```python
from build123d import *

# Parameters (mm, degrees)
F0_R     = 3.2639
F0_R_2   = 14.224
F1_DEPTH = 12.7
F2_R     = 6.35


# Not quite as in the source:
# - ends of sketch curves that miss each other by under 0.0002 mm in the source are joined


with BuildPart() as f1:
    # F0 (on Top) → F1 (new body)
    with BuildSketch(Plane.XY):
        with BuildLine():
            Line((-19.0499999385, -12.7), (19.0500000615, -12.7))
            ThreePointArc((19.0500000615, -12.7), (23.5401281437, -10.8401280388), (25.4000000615, -6.3499999385))
            Line((25.4000000615, -6.3499999385), (25.3999998771, 12.7))
            Line((25.3999998771, 12.7), (20.257849715, 41.692909813))
            ThreePointArc((20.257849715, 41.692909813), (0, 58.674), (-20.257849715, 41.692909813))
            Line((-20.257849715, 41.692909813), (-25.4000001229, 12.7))
            Line((-25.4000001229, 12.7), (-25.3999999385, -6.3500000615))
            ThreePointArc((-25.3999999385, -6.3500000615), (-23.5401279774, -10.8401280823), (-19.0499999385, -12.7))
        make_face()
        with Locations((-16.256, 0)):
            Circle(F0_R, mode=Mode.SUBTRACT)
        with Locations((15.494, 0)):
            Circle(F0_R, mode=Mode.SUBTRACT)
        with Locations((0, 38.1)):
            Circle(F0_R_2, mode=Mode.SUBTRACT)
    extrude(amount=F1_DEPTH)

    # F2
    f2_edges = [f1.edges().sort_by_distance(p)[0] for p in [
        (25.4, 12.7, 6.35),
        (-25.4, 12.7, 6.35),
    ]]
    fillet(f2_edges, radius=F2_R)


solid = f1.part
```
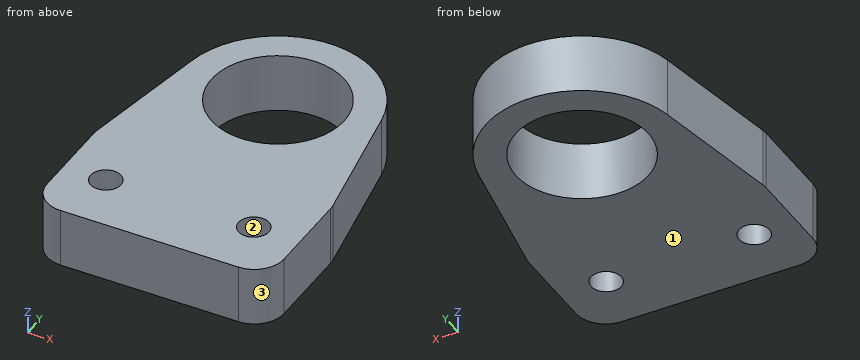
Part model, mm, in its own coordinate system. Face numbers are marked on the shaded views. Round coordinates to 2 decimals unless told otherwise and drop trailing zeros. Write each loop counter-clockwise with the first axis right and the second up, starting at its lowest first coordinate (ties: lowest second). Pieces come first, ordered by that corner, then holes.
Item 1: Probe L1, parallel to X at y = -1, z = 2.25; L2, parallel to Y at x = 0, z = 5.25; L3, parallel to X at y = 49, z = 12. List the from-to ranges inside material, lowest first.
Results:
L1: x = -25.4 to -19.36, -13.15 to 12.39, 18.6 to 25.4
L2: y = -12.7 to 23.88, 52.32 to 58.67
L3: x = -17.45 to -9.14, 9.14 to 17.45
Item 2: Cut at B-B, the plane x = 0. Give the cut face in (y, z).
Results:
outline: (-12.7, 0) - (23.88, 0) - (23.88, 12.7) - (-12.7, 12.7) - close; (52.32, 0) - (58.67, 0) - (58.67, 12.7) - (52.32, 12.7) - close
Item 3: Cut at C-C, the plane z = 6.5. Give the cut face in (x, y).
Results:
outline: (-25.4, -6.35) arc R6.35 ccw to (-19.05, -12.7) - (19.05, -12.7) arc R6.35 ccw to (25.4, -6.35) - (25.4, 12.14) arc R6.35 ccw to (25.3, 13.25) - (20.26, 41.69) arc R20.57 ccw to (-20.26, 41.69) - (-25.3, 13.25) arc R6.35 ccw to (-25.4, 12.14) - close; hole circle Ø6.53 at (-16.26, 0); hole circle Ø28.45 at (0, 38.1); hole circle Ø6.53 at (15.49, 0)
Item 4: Cut at D-D, the plane y = 26. Give the cut face in (x, z).
Results:
outline: (-23.04, 0) - (-7.48, 0) - (-7.48, 12.7) - (-23.04, 12.7) - close; (7.48, 0) - (23.04, 0) - (23.04, 12.7) - (7.48, 12.7) - close
Item 5: Cut at A-A, the plane y = 0. Give the cut face in (x, z).
Results:
outline: (-25.4, 0) - (-19.52, 0) - (-19.52, 12.7) - (-25.4, 12.7) - close; (-12.99, 0) - (12.23, 0) - (12.23, 12.7) - (-12.99, 12.7) - close; (18.76, 0) - (25.4, 0) - (25.4, 12.7) - (18.76, 12.7) - close
Item 6: Drop flat-ended pins along their axis: pin 1 Ø4 at (y, z) = (39, 5) entering from -X; pin 2 Ø5 at (y, z) = (24, 4.5) entering from -X; pin 3 Ø1 at (x, z) = (-2, 5) entering from +Y. Give the stop position or say it passes through.
Results:
pin 1: stops at x = -21.09
pin 2: stops at x = -23.84
pin 3: stops at y = 58.62
Item 7: Two-plate mould, pull along X, no slides. Class the marked faces 1, 2 and 3: +X half, -X half, draft (parallel to the pull), parting line (faces both ways), or undercut.
Results:
face 1: draft
face 2: undercut
face 3: +X half
